Part model, mm, in its own coordinate system. A direction names the side the tool comes from. Give positions to 0.01 mm unless a question says otherwise; leave off trailing zeros. Write each loop counter-clockwise with the first axis right and the second up, starting at its lowest first coordinate (ties: lowest second). Pieces come first, ordered by that corner, then holes.
from build123d import *

# Parameters (mm, degrees)
CROQUIS1_W              = 13
CROQUIS1_H              = 1
CROQUIS1_W_2            = 1
CROQUIS1_H_2            = 13
SALIENTE_EXTRUIR1_DEPTH = 400
CROQUIS2_R              = 2.38125
CORTAR_EXTRUIR1_DEPTH   = 10
CROQUIS3_R              = 2.38125
CORTAR_EXTRUIR2_DEPTH   = 10


with BuildPart() as part:
    # Croquis1 → Saliente-Extruir1 (new body, symmetric)
    with BuildSketch(Plane.XY):
        with BuildLine():
            ThreePointArc((-13.7, 13.681053808), (5.967619023, 5.967619023), (13.681053808, -13.7))
            Line((13.681053808, -13.7), (-13.7, -13.7))
            Line((-13.7, -13.7), (-13.7, 13.681053808))
        make_face()
        with BuildLine():
            Line((-12.7, -12.7), (-12.7, 12.7))
            ThreePointArc((-12.7, 12.7), (5.260512242, 5.260512242), (12.7, -12.7))
            Line((12.7, -12.7), (-12.7, -12.7))
        make_face(mode=Mode.SUBTRACT)
        with Locations((-20.2, 13.181053808)):
            Rectangle(CROQUIS1_W, CROQUIS1_H)
        with Locations((13.181053808, -20.2)):
            Rectangle(CROQUIS1_W_2, CROQUIS1_H_2)
    extrude(amount=SALIENTE_EXTRUIR1_DEPTH, both=True)

    # Croquis2 → Cortar-Extruir1 (cut)
    with BuildSketch(Plane(origin=(0, 13.681053808, 0), x_dir=(1, 0, 0), z_dir=(0, 1, 0))):
        with Locations((-18.7, -210.5)):
            Circle(CROQUIS2_R)
        with Locations((-18.7, -229.5)):
            Circle(CROQUIS2_R)
        with Locations((-18.7, 229.5)):
            Circle(CROQUIS2_R)
        with Locations((-18.7, 210.5)):
            Circle(CROQUIS2_R)
    extrude(amount=-CORTAR_EXTRUIR1_DEPTH, mode=Mode.SUBTRACT)

    # Croquis3 → Cortar-Extruir2 (cut)
    with BuildSketch(Plane(origin=(13.681053808, 0, 0), x_dir=(0, 0, -1), z_dir=(1, 0, 0))):
        with Locations((-229.5, -21.7)):
            Circle(CROQUIS3_R)
        with Locations((-210.5, -21.7)):
            Circle(CROQUIS3_R)
        with Locations((210.5, -21.7)):
            Circle(CROQUIS3_R)
        with Locations((229.5, -21.7)):
            Circle(CROQUIS3_R)
    extrude(amount=-CORTAR_EXTRUIR2_DEPTH, mode=Mode.SUBTRACT)


solid = part.part
1) 3-axis set-ups, long thin cutter, end or side, ignore diameter. For faces 1 (the flat face through (13.681, -20, 6)), 2 (the flat face through (0, -12.7, 6)), 3 (the flat face through (-20, 12.681, 6)): which of +Z, -Z, +X, -X, +Y, -Y reach the whole face in a straight line?
Check result:
face 1: +Z, -Z, +X, +Y, -Y
face 2: +Z, -Z
face 3: +Z, -Z, -X, -Y
2) Saw through at C-C (y = 4). Write the cut outline in (x, z).
Check result:
outline: (-13.7, -400) - (-12.7, -400) - (-12.7, 400) - (-13.7, 400) - close; (6.44, -400) - (7.75, -400) - (7.75, 400) - (6.44, 400) - close
3) Saw through at B-B (x = -2). Write the cut outline in (y, z).
Check result:
outline: (-13.7, -400) - (-12.7, -400) - (-12.7, 400) - (-13.7, 400) - close; (10.34, -400) - (11.43, -400) - (11.43, 400) - (10.34, 400) - close
4) Flat gauge pins, fed straight in: P1, Ø8, axis at x = -5, z = 108.5, coming from the +Y side; P2, Ø8, axis at x = -4, z = -27.5, coming from the +Y side; P3, Ø5, axis at x = 7, z = -56, coming from the -Y side. Where does each tip first touch, or does it go through?
Check result:
P1: stops at y = 13.44
P2: stops at y = 13.28
P3: stops at y = -13.7
5) Drill centre lines: L1, parallel to Z at x = 13, y = -21; L2, parallel to Z at x = -18.7, y = 13.45; L3, parallel to X at y = -10.5, z = -106.5. Where is each one in solid material? Low to high.
Check result:
L1: z = -400 to -231.78, -227.22 to -212.78, -208.22 to 208.22, 212.78 to 227.22, 231.78 to 400
L2: z = -400 to -231.88, -227.12 to -212.88, -208.12 to 208.12, 212.88 to 227.12, 231.88 to 400
L3: x = -13.7 to -12.7, 12.6 to 13.61
6) Mould opens along Y. For faces 4 (the flat face through (-12.7, 0, 6)), 5 (the cylindrical face through (5.06, 5.46, 5.6)), 6 (the flat face through (5.6, 5.6, 400)), 7 (the flat face through (-20, 13.681, 6)) say: +Y half, -Y half, draft (parallel to the pull), parting line (faces both ways), or undercut.
Check result:
face 4: undercut
face 5: undercut
face 6: draft
face 7: +Y half
7) Saw through at A-A (z = -323.5). Write the cut outline in (x, y).
Check result:
outline: (-26.7, 12.68) - (-13.7, 12.68) - (-13.7, -13.7) - (12.68, -13.7) - (12.68, -26.7) - (13.68, -26.7) - (13.68, -13.7) arc R26.4 ccw to (-13.7, 13.68) - (-26.7, 13.68) - close; hole (-12.7, -12.7) - (12.7, -12.7) arc R25.4 ccw to (-12.7, 12.7) - close
